Autodesk Inventor part; units mm, degrees
ref_plane "YZ Plane" through (0, 0, 0) normal (1, 0, 0) x (0, 1, 0)
ref_plane "XZ Plane" through (0, 0, 0) normal (0, 1, 0) x (-1, 0, 0)
ref_plane "XY Plane" through (0, 0, 0) normal (0, 0, 1) x (1, 0, 0)
sketch "Sketch1" plane through (0, 0, 0) normal (0, 1, 0) x (-1, 0, 0)
  line L0 (0, 0) -> (-130, 0)
  line L1 (-130, 0) -> (-130, 20)
  line L2 (-130, 20) -> (0, 20)
  line L3 (0, 20) -> (0, 0)
  dimension "d0" = 130
  dimension "d1" = 20
extrude "Extrusion1" add sketch "Sketch1" along normal blind 2
hole "Hole1" at (12, 2, 10) direction (0, -1, 0) diameter 5.5 end through all
pattern_linear "Rectangular Pattern1" count 2 spacing 103.172 along (1, 0, 0) of "Hole1"
properties part number "lastflat bar" material "Aluminum 6061"
Source: CAD feature listing. Evaluate the final solid. Frame: model axes, mm. Round coordinates to 2 decimals unless told otherwise and drop trailing zeros. Loops run counter-clockwise (first coordinate to the right, second up) from the corner with the lowest first, then second, coordinate; pieces in that order, holes last.
1. Ray query, L1, parallel to X at y = 1.25, z = 10; L2, parallel to Z at x = 12, y = 0.7; L3, parallel to X at y = 1.1, z = 8. Return the intervals inside material, ascending.
2. Section query C-C on y = 0.9. Output: boundary loops of the cut face in (x, z).
3. Contact query for a flat-ended pin moving along its axis: pin 1 (4.5 mm diameter, centred on x = 12, z = 10, fed in from -Y). Output: stop coordinate, or through.
4. Section query A-A on z = 10. Output: boundary loops of the cut face in (x, y), and give its area (3 significant figures).
5. Mould query, pull axis Z, two halves, no side actions, for faces 1 (the cylindrical face through (112.853, 0.986, 11.478)), 2 (the flat face through (64, 1, 0)), 3 (the flat face through (66, 0, 10)). Classes: released by +Z, released by -Z, zero draft, split by the parting line, or undercut.
6. Section query B-B on x = 12. Output: boundary loops of the cut face in (y, z).
Answers below:
1. L1: x = 0 to 9.25, 14.75 to 112.42, 117.92 to 130
1. L2: z = 0 to 7.25, 12.75 to 20
1. L3: x = 0 to 10.11, 13.89 to 113.28, 117.06 to 130
2. outline: (0, 0) - (130, 0) - (130, 20) - (0, 20) - close; hole circle Ø5.5 at (12, 10); hole circle Ø5.5 at (115.17, 10)
3. pin 1: passes through
4. outline: (0, 0) - (9.25, 0) - (9.25, 2) - (0, 2) - close; (14.75, 0) - (112.42, 0) - (112.42, 2) - (14.75, 2) - close; (117.92, 0) - (130, 0) - (130, 2) - (117.92, 2) - close
4. area: 238 mm2
5. face 1: undercut
5. face 2: released by -Z
5. face 3: zero draft
6. outline: (0, 0) - (2, 0) - (2, 7.25) - (0, 7.25) - close; (0, 12.75) - (2, 12.75) - (2, 20) - (0, 20) - close
